CAD build for the part. Positions are in the model's coordinates, mm. Face numbers are marked on the shaded views. A direction names the side the tool comes from. Round coordinates to 2 decimals unless told otherwise and drop trailing zeros. Loops run counter-clockwise (first coordinate to the right, second up) from the corner with the lowest first, then second, coordinate; pieces in that order, holes last. Notation, with made-up numbers: M -37.5,-14 L 16.5,-14 A19 ccw 16.5,-3 Z; hole C -23.5,51.5 d8. An arc over 180 degrees is marked long. Put each result on its own line as item: value. Start each with the question number.
from build123d import *

# Parameters (mm, degrees)
SKETCH1_W                = 45.3
SKETCH1_H                = 65.4
BOSS_EXTRUDE1_DEPTH      = 3
BOSS_EXTRUDE2_DEPTH      = 27.25
BOSS_EXTRUDE3_START      = -32.7
BOSS_EXTRUDE3_DEPTH      = 65.4
CUT_EXTRUDE1_DEPTH       = 65.254280101
CUT_EXTRUDE1_DEPTH_BACK  = 65.254280101
CUT_EXTRUDE3_DEPTH       = 15.325997
BOSS_EXTRUDE4_START      = 6
BOSS_EXTRUDE4_DEPTH      = 6
CUT_EXTRUDE4_DEPTH       = 92.386822264
BOSS_EXTRUDE5_DEPTH      = 92.9
BOSS_EXTRUDE5_DEPTH_BACK = 92.9
BOSS_EXTRUDE6_DEPTH      = 60.2
BOSS_EXTRUDE7_START      = 2
BOSS_EXTRUDE7_DEPTH      = 2
BOSS_EXTRUDE8_START      = -63.2
BOSS_EXTRUDE8_DEPTH      = 123.4


# Read off the part's stored shape, not the designer's step: Boss-Extrude3
with BuildPart() as part:
    # Sketch1 → Boss-Extrude1 (new, symmetric)
    with BuildSketch(Plane.XY):
        Rectangle(SKETCH1_W, SKETCH1_H)
        with BuildLine():
            Line((3, 27.5), (3, -27.5))
            ThreePointArc((3, -27.5), (0, -30.5), (-3, -27.5))
            Line((-3, -27.5), (-3, 27.5))
            ThreePointArc((-3, 27.5), (0, 30.5), (3, 27.5))
        make_face(mode=Mode.SUBTRACT)
    extrude(amount=BOSS_EXTRUDE1_DEPTH, both=True)

    # Sketch3 → Boss-Extrude2 (add)
    with BuildSketch(Plane(origin=(0, 0, -3), x_dir=(-1, 0, 0), z_dir=(0, 0, -1))):
        with BuildLine():
            Line((4.65, 28.050000345), (4.65, -28.050000676))
            ThreePointArc((4.65, -28.050000676), (0, -32.7), (-4.65, -28.050000677))
            Line((-4.65, -28.050000677), (-4.65, 28.050000345))
            ThreePointArc((-4.65, 28.050000345), (0, 32.7), (4.65, 28.050000345))
        make_face()
    extrude(amount=BOSS_EXTRUDE2_DEPTH)

    # Boss-Extrude3 outline → Boss-Extrude3 (add)
    with BuildSketch(Plane(origin=(0, 0, 0), x_dir=(1, 0, 0), z_dir=(0, 1, 0)).offset(BOSS_EXTRUDE3_START)):
        with BuildLine():
            Line((4.65, 31.477081959), (4.65, 46.803079293))
            ThreePointArc((4.65, 46.803079293), (14.382164808, 45.086281989), (23.65, 41.655588809))
            Line((23.65, 41.655588809), (23.65, 44.959205999))
            ThreePointArc((23.65, 44.959205999), (0, 50), (-23.65, 44.959205999))
            Line((-23.65, 44.959205999), (-23.65, 41.655588809))
            ThreePointArc((-23.65, 41.655588809), (-14.382164808, 45.086281989), (-4.65, 46.803079293))
            Line((-4.65, 46.803079293), (-4.65, 31.477081959))
            ThreePointArc((-4.65, 31.477081959), (-14.64207711, 28.955000716), (-23.65, 23.949021894))
            Line((-23.65, 23.949021894), (-23.65, 22.06226871))
            ThreePointArc((-23.65, 22.06226871), (-12.513607029, 28.145153743), (3e-09, 30.25))
            ThreePointArc((3e-09, 30.25), (12.513607029, 28.145153743), (23.65, 22.06226871))
            Line((23.65, 22.06226871), (23.65, 23.949021894))
            ThreePointArc((23.65, 23.949021894), (14.64207711, 28.955000716), (4.65, 31.477081959))
        make_face()
    extrude(amount=BOSS_EXTRUDE3_DEPTH)

    # Sketch5 → Cut-Extrude1 (cut, two sides: drawn at the far end of the back side and taken through both)
    with BuildSketch(Plane.XY.offset(-CUT_EXTRUDE1_DEPTH_BACK)):
        with BuildLine():
            Line((3, -27.5), (3, 27.5))
            ThreePointArc((3, 27.5), (0, 30.5), (-3, 27.5))
            Line((-3, 27.5), (-3, -27.5))
            ThreePointArc((-3, -27.5), (0, -30.5), (3, -27.5))
        make_face()
    extrude(amount=CUT_EXTRUDE1_DEPTH + CUT_EXTRUDE1_DEPTH_BACK, mode=Mode.SUBTRACT)

    # Sketch6 → Cut-Extrude3 (cut)
    with BuildSketch(Plane(origin=(0, 0, -31.477081959), x_dir=(-1, 0, 0), z_dir=(0, 0, -1))):
        with BuildLine():
            ThreePointArc((0, -32.7), (-3.288046293, -31.338046772), (-4.65, -28.050000677))
            Line((-4.65, -28.050000677), (-4.65, -32.7))
            Line((-4.65, -32.7), (0, -32.7))
        make_face()
        with BuildLine():
            ThreePointArc((4.65, -28.050000676), (3.288046294, -31.338046771), (0, -32.7))
            Line((0, -32.7), (4.65, -32.7))
            Line((4.65, -32.7), (4.65, -28.050000676))
        make_face()
        with BuildLine():
            Line((-4.65, 32.7), (-4.65, 28.050000345))
            ThreePointArc((-4.65, 28.050000345), (-3.288046411, 31.338046654), (0, 32.7))
            Line((0, 32.7), (-4.65, 32.7))
        make_face()
        with BuildLine():
            Line((4.65, 32.7), (0, 32.7))
            ThreePointArc((0, 32.7), (3.28804641, 31.338046655), (4.65, 28.050000345))
            Line((4.65, 28.050000345), (4.65, 32.7))
        make_face()
    extrude(amount=CUT_EXTRUDE3_DEPTH, mode=Mode.SUBTRACT)

    # Sketch8 → Boss-Extrude4 (add)
    with BuildSketch(Plane(origin=(0, -29.7, 0), x_dir=(-1, 0, 0), z_dir=(0, -1, 0)).offset(BOSS_EXTRUDE4_START)):
        with BuildLine():
            ThreePointArc((23.65, 44.959205999), (0, 50), (-23.65, 44.959205999))
            Line((-23.65, 44.959205999), (-23.65, 46.959205999))
            ThreePointArc((-23.65, 46.959205999), (0, 51.906346228), (23.65, 46.959205999))
            Line((23.65, 46.959205999), (23.65, 44.959205999))
        make_face()
    boss_extrude4 = extrude(amount=-BOSS_EXTRUDE4_DEPTH)

    # Mirror1: Boss-Extrude4 across plane
    add(boss_extrude4.mirror(Plane.ZX))

    # Sketch10 → Cut-Extrude4 (cut, through all)
    with BuildSketch(Plane(origin=(0, 35.7, 0), x_dir=(1, 0, 0), z_dir=(0, 1, 0))):
        with BuildLine():
            ThreePointArc((0, 51.906346228), (-2.389460165, 51.857943444), (-4.775, 51.712814503))
            Line((-4.775, 51.712814503), (-4.775, 49.803108697))
            ThreePointArc((-4.775, 49.803108697), (-2.389528781, 49.950756269), (0, 50))
            Line((0, 50), (0, 51.906346228))
        make_face()
        with BuildLine():
            ThreePointArc((4.775, 51.712814503), (2.389460165, 51.857943444), (0, 51.906346228))
            Line((0, 51.906346228), (0, 50))
            ThreePointArc((0, 50), (2.389528781, 49.950756269), (4.775, 49.803108697))
            Line((4.775, 49.803108697), (4.775, 51.712814503))
        make_face()
        with BuildLine():
            ThreePointArc((-4.775, 51.712814503), (-4.925016027, 51.700441497), (-5.075, 51.687685822))
            Line((-5.075, 51.687685822), (-5.075, 49.777542134))
            ThreePointArc((-5.075, 49.777542134), (-4.92501659, 49.790520084), (-4.775, 49.803108697))
            Line((-4.775, 49.803108697), (-4.775, 51.712814503))
        make_face()
        with BuildLine():
            ThreePointArc((5.075, 51.687685822), (4.925016027, 51.700441497), (4.775, 51.712814503))
            Line((4.775, 51.712814503), (4.775, 49.803108697))
            ThreePointArc((4.775, 49.803108697), (4.92501659, 49.790520084), (5.075, 49.777542134))
            Line((5.075, 49.777542134), (5.075, 51.687685822))
        make_face()
    extrude(amount=-CUT_EXTRUDE4_DEPTH, mode=Mode.SUBTRACT)

    # Sketch11 → Boss-Extrude5 (add, two sides: drawn at the far end of the back side and taken through both)
    with BuildSketch(Plane(origin=(0, 0, 0), x_dir=(1, 0, 0), z_dir=(0, 1, 0)).offset(-BOSS_EXTRUDE5_DEPTH_BACK)):
        with BuildLine():
            ThreePointArc((-5.575, 49.731441823), (-5.325049888, 49.755033059), (-5.075, 49.777542134))
            Line((-5.075, 49.777542134), (-5.075, 51.787685822))
            Line((-5.075, 51.787685822), (-2.55, 51.787685822))
            Line((-2.55, 51.787685822), (-2.55, 52.287685822))
            Line((-2.55, 52.287685822), (-5.575, 52.287685822))
            Line((-5.575, 52.287685822), (-5.575, 49.731441823))
        make_face()
        with BuildLine():
            ThreePointArc((5.075, 49.777542134), (5.325049888, 49.755033059), (5.575, 49.731441823))
            Line((5.575, 49.731441823), (5.575, 52.287685822))
            Line((5.575, 52.287685822), (2.55, 52.287685822))
            Line((2.55, 52.287685822), (2.55, 51.787685822))
            Line((2.55, 51.787685822), (5.075, 51.787685822))
            Line((5.075, 51.787685822), (5.075, 49.777542134))
        make_face()
    extrude(amount=BOSS_EXTRUDE5_DEPTH + BOSS_EXTRUDE5_DEPTH_BACK)

    # Sketch13 → Boss-Extrude6 (add)
    with BuildSketch(Plane(origin=(0, -92.9, 0), x_dir=(-1, 0, 0), z_dir=(0, -1, 0))):
        with BuildLine():
            ThreePointArc((-5.075, 49.777542134), (-5.325049888, 49.755033059), (-5.575, 49.731441823))
            Line((-5.575, 49.731441823), (-5.575, 47.219284448))
            ThreePointArc((-5.575, 47.219284448), (-5.123234459, 47.263029854), (-4.671126278, 47.303079293))
            Line((-4.671126278, 47.303079293), (0, 47.303079293))
            Line((0, 47.303079293), (4.671126278, 47.303079293))
            ThreePointArc((4.671126278, 47.303079293), (5.123234459, 47.263029854), (5.575, 47.219284448))
            Line((5.575, 47.219284448), (5.575, 49.731441823))
            ThreePointArc((5.575, 49.731441823), (5.325049888, 49.755033059), (5.075, 49.777542134))
            ThreePointArc((5.075, 49.777542134), (0, 50), (-5.075, 49.777542134))
        make_face()
    extrude(amount=-BOSS_EXTRUDE6_DEPTH)

    # Sketch14 → Boss-Extrude7 (add)
    with BuildSketch(Plane(origin=(0, -92.9, 0), x_dir=(-1, 0, 0), z_dir=(0, -1, 0)).offset(BOSS_EXTRUDE7_START)):
        with BuildLine():
            Line((-2.55, 52.287685822), (2.55, 52.287685822))
            Line((2.55, 52.287685822), (5.575, 52.287685822))
            Line((5.575, 52.287685822), (5.575, 47.219284448))
            ThreePointArc((5.575, 47.219284448), (5.123234459, 47.263029854), (4.671126278, 47.303079293))
            Line((4.671126278, 47.303079293), (-4.671126278, 47.303079293))
            ThreePointArc((-4.671126278, 47.303079293), (-5.123234459, 47.263029854), (-5.575, 47.219284448))
            Line((-5.575, 47.219284448), (-5.575, 52.287685822))
            Line((-5.575, 52.287685822), (-2.55, 52.287685822))
        make_face()
    extrude(amount=-BOSS_EXTRUDE7_DEPTH)

    # Sketch15 → Boss-Extrude8 (add)
    with BuildSketch(Plane(origin=(0, 32.7, 0), x_dir=(1, 0, 0), z_dir=(0, 1, 0)).offset(BOSS_EXTRUDE8_START)):
        with BuildLine():
            ThreePointArc((-5.075, 49.777542134), (-5.325049888, 49.755033059), (-5.575, 49.731441823))
            Line((-5.575, 49.731441823), (-5.575, 48.726707775))
            ThreePointArc((-5.575, 48.726707775), (0, 49), (5.575, 48.726707775))
            Line((5.575, 48.726707775), (5.575, 49.731441823))
            ThreePointArc((5.575, 49.731441823), (5.325049888, 49.755033059), (5.075, 49.777542134))
            ThreePointArc((5.075, 49.777542134), (0, 50), (-5.075, 49.777542134))
        make_face()
    boss_extrude8 = extrude(amount=BOSS_EXTRUDE8_DEPTH)

    # Mirror2: Boss-Extrude8 across plane
    add(boss_extrude8.mirror(Plane.ZX))


solid = part.part
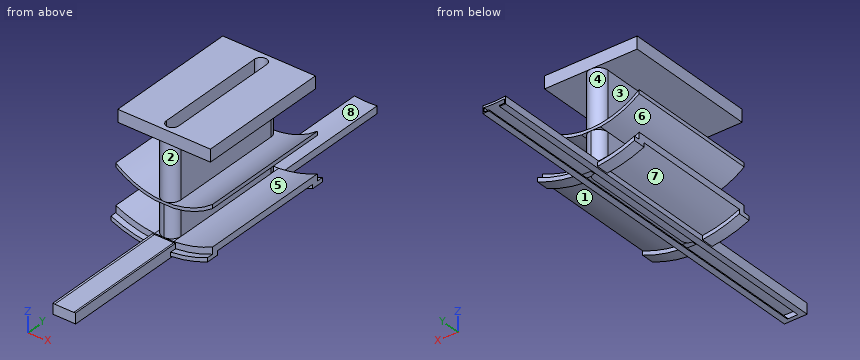
(1) Cut at A-A on x = -16. List the corners of the cut face in (y, z), and give its area (3 significant figures).
(2) Tool access for the marked faces 5, 6, 7 and 8: list every direction of +Z, -Z, +X, -X, +Y, -Y with a clear straight run to the whole face (end or side of a thin tool).
(3) Drill centre lines: line 1 along Z through (x, y) = (17, -30); line 2 along Z through (x, y) = (-21, 2.5); line 3 along X through (y, z) = (28, -42.5). Where is each one in solid material? Low to high.
(4) Flat gauge pins, fed straight in: pin 1 Ø3 at (y, z) = (8, -0.5) entering from -X; pin 2 Ø1.8 at (x, z) = (4.5, 0) entering from +Y; pin 3 Ø4 at (y, z) = (-30.5, -49.5) entering from -X. Where does each tip first touch, or does it go through?
(5) Cut at C-C on y = 52. List the corners of the cut face in (x, z) (3 decimals).
(6) Cut at B-B on z = -28. List the corners of the cut face in (x, y).
(7) Cut at D-D on x = -7.5. List the corners of the cut face in (y, z), and give its area (3 significant figures).
(8) Mould opens along Y. For the marked faces 1, 2, 3 and 4 say: +Y half, -Y half, draft (parallel to the pull), parting line (faces both ways), or undercut.
Taken from the geometry:
1. outline: M -35.7,-49.7 L -29.7,-49.7 L -29.7,-47.75 L 29.7,-47.75 L 29.7,-49.7 L 35.7,-49.7 L 35.7,-47.75 L 32.7,-47.75 L 32.7,-44.62 L -32.7,-44.62 L -32.7,-47.75 L -35.7,-47.75 Z; M -32.7,-28.39 L 32.7,-28.39 L 32.7,-26.74 L -32.7,-26.74 Z; M -32.7,-3 L 32.7,-3 L 32.7,3 L -32.7,3 Z
1. area: 728 mm2
2. face 5: +Y, -Y
2. face 6: -X, +Y, -Y
2. face 7: -Z, -X
2. face 8: +Z, +Y
3. line 1: -49.4 to -44.31, -27.93 to -26.26, -3 to 3
3. line 2: -46.06 to -42.83, -25.75 to -23.97, -3 to 3
3. line 3: -23.65 to -21.79, -4.65 to -2.96, 2.96 to 4.65, 21.79 to 23.65
4. pin 1: x = -22.65
4. pin 2: y = 32.7
4. pin 3: x = -22.37
5. outline: M -5.575,-52.288 L -2.55,-52.288 L -2.55,-51.788 L -5.075,-51.788 L -5.075,-49.778 A58 ccw 5.075,-49.778 L 5.075,-51.788 L 2.55,-51.788 L 2.55,-52.288 L 5.575,-52.288 L 5.575,-48.727 A57 cw -5.575,-48.727 Z
6. outline: M -16.85,-32.7 L -12.93,-32.7 L -12.93,32.7 L -16.85,32.7 Z; M -4.65,-28.05 A4.65 ccw 4.65,-28.05 L 4.65,28.05 A4.65 ccw -4.65,28.05 Z; M 12.93,-32.7 L 16.85,-32.7 L 16.85,32.7 L 12.93,32.7 Z; hole M -3,-27.5 A3 ccw 3,-27.5 L 3,27.5 A3 ccw -3,27.5 Z
7. outline: M -35.7,-51.43 L -29.7,-51.43 L -29.7,-49.51 L 29.7,-49.51 L 29.7,-51.43 L 35.7,-51.43 L 35.7,-49.51 L 32.7,-49.51 L 32.7,-46.49 L -32.7,-46.49 L -32.7,-49.51 L -35.7,-49.51 Z; M -32.7,-31.04 L 32.7,-31.04 L 32.7,-29.51 L -32.7,-29.51 Z; M -32.7,-3 L 32.7,-3 L 32.7,3 L -32.7,3 Z
7. area: 713 mm2
8. face 1: undercut
8. face 2: -Y half
8. face 3: draft
8. face 4: +Y half
